Source: three-view drawing plus pictorial views. Frame: mm from the lowest corner of the part. A direction names the side the tool comes from. Coordinates: 2 decimals unless noted, no trailing zeros. Write each loop counter-clockwise with the first axis right and the second up, starting at its lowest first coordinate (ties: lowest second). Pieces come first, ordered by that corner, then holes. Notation, with made-up numbers: (-38, 39) - (-31, 39) arc R7 ccw to (-31, 45) - close; hole circle Ø5 at (-33.5, 54.25). An arc over 180 degrees is marked (long way). One line per item, written item: value.
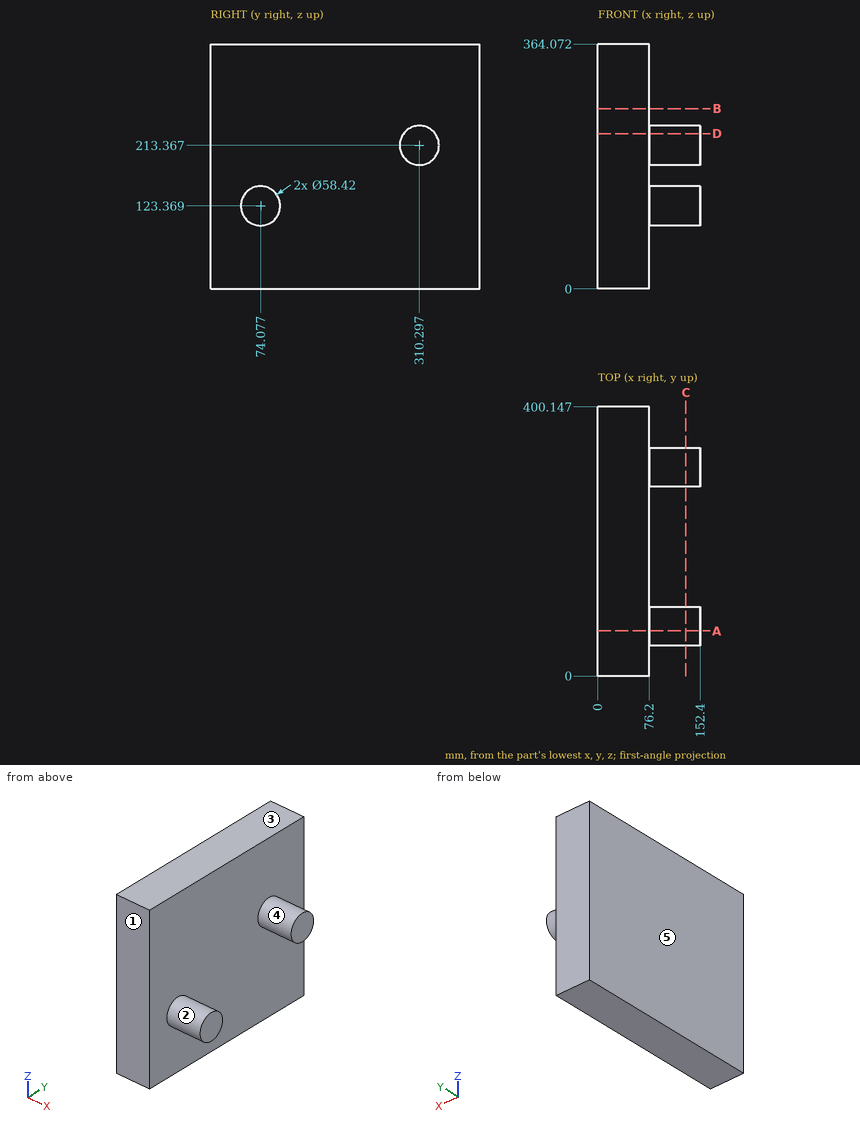
1) Section query A-A on y = 67. Output: boundary loops of the cut face in (x, z), then the cut area to 3 significant figures.
Values found:
outline: (0, 0) - (76.2, 0) - (76.2, 95.03) - (152.4, 95.03) - (152.4, 151.71) - (76.2, 151.71) - (76.2, 364.07) - (0, 364.07) - close
area: 32,100 mm2
2) Section query C-C on x = 131. Output: boundary loops of the cut face in (y, z), then the cut area to 3 significant figures.
Values found:
outline: circle Ø58.42 at (74.08, 123.37); circle Ø58.42 at (310.3, 213.37)
area: 5,360 mm2
3) Draft query along Y for the marked faces 1, 2 and 3. Return one class per face: released by +Y, released by -Y, zero draft, split by the parting line, or undercut.
Values found:
face 1: released by -Y
face 2: split by the parting line
face 3: zero draft
4) Material intervals for line 1 (X direction, y = 34, z = 217.5); line 2 (Y direction, x = 78, z = 212) (1 decimal); line 3 (Y direction, x = 141.5, z = 139), sorted ascending.
Values found:
line 1: 0 to 76.2
line 2: 281.1 to 339.5
line 3: 49.4 to 98.75
5) Section query D-D on z = 231. Output: boundary loops of the cut face in (x, y) (1 decimal).
Values found:
outline: (0, 0) - (76.2, 0) - (76.2, 287) - (152.4, 287) - (152.4, 333.6) - (76.2, 333.6) - (76.2, 400.1) - (0, 400.1) - close
6) Section query B-B on z = 268. Output: boundary loops of the cut face in (x, y), then the cut area to 3 significant figures.
Values found:
outline: (0, 0) - (76.2, 0) - (76.2, 400.15) - (0, 400.15) - close
area: 30,500 mm2
7) Reachability of the marked faces 4 and 5 from +Z, -Z, +X, -X, +Y, -Y: full face, straight path, thin tool, end or side. Return the list, or none.
Values found:
face 4: +X
face 5: +Z, -Z, -X, +Y, -Y
8) Contact query for flat-ended pins moving along their axis: P1, Ø1, axis at y = 301.5, z = 138, coming from the +X side; P2, Ø6, axis at x = 84, y = 312.5, coming from the +Z side. Output: stop coordinate, or through.
Values found:
P1: x = 76.2
P2: z = 242.58
